from build123d import *

# Parameters (mm, degrees)
SKETCH1_W           = 170
SKETCH1_H           = 216
BOSS_EXTRUDE1_DEPTH = 5
SKETCH2_R           = 1.5
CUT_EXTRUDE1_DEPTH  = 138.528178931
SKETCH9_W           = 170
SKETCH9_H           = 90
BOSS_EXTRUDE2_DEPTH = 3
SKETCH10_W          = 219
SKETCH10_H          = 90
BOSS_EXTRUDE3_DEPTH = 5
BOSS_EXTRUDE5_START = 5
SKETCH11_W          = 219
SKETCH11_H          = 90
BOSS_EXTRUDE5_DEPTH = 5
SKETCH14_W          = 180
SKETCH14_H          = 90
CUT_EXTRUDE2_DEPTH  = 3
SKETCH15_W          = 180
SKETCH15_H          = 90
BOSS_EXTRUDE6_DEPTH = 5


with BuildPart() as part:
    # Sketch1 → Boss-Extrude1 (new body)
    with BuildSketch(Plane(origin=(0, 0, 0), x_dir=(1, 0, 0), z_dir=(0, 1, 0))):
        Rectangle(SKETCH1_W, SKETCH1_H)
    extrude(amount=BOSS_EXTRUDE1_DEPTH)

    # Sketch2 → Cut-Extrude1 (cut, through all)
    with BuildSketch(Plane(origin=(0, 5, 0), x_dir=(1, 0, 0), z_dir=(0, 1, 0))):
        with Locations(Location((-75, 98, 0), (0, 0, 270))):
            Circle(SKETCH2_R)
        with Locations(Location((75, 98, 0), (0, 0, 270))):
            Circle(SKETCH2_R)
        with Locations(Location((-75, -98, 0), (0, 0, 270))):
            Circle(SKETCH2_R)
        with Locations(Location((75, -98, 0), (0, 0, 270))):
            Circle(SKETCH2_R)
    extrude(amount=-CUT_EXTRUDE1_DEPTH, mode=Mode.SUBTRACT)

    # Sketch9 → Boss-Extrude2 (add)
    with BuildSketch(Plane(origin=(0, 0, -108), x_dir=(-1, 0, 0), z_dir=(0, 0, -1))):
        with Locations((0, 45)):
            Rectangle(SKETCH9_W, SKETCH9_H)
    extrude(amount=BOSS_EXTRUDE2_DEPTH)

    # Sketch10 → Boss-Extrude3 (add)
    with BuildSketch(Plane(origin=(85, 0, 0), x_dir=(0, 0, -1), z_dir=(1, 0, 0))):
        with Locations((1.5, 45)):
            Rectangle(SKETCH10_W, SKETCH10_H)
        with BuildLine():
            Line((-84, 5), (-41, 5))
            Line((-41, 5), (-41, 44))
            ThreePointArc((-41, 44), (-41.878679656, 46.121320344), (-44, 47))
            Line((-44, 47), (-81, 47))
            ThreePointArc((-81, 47), (-83.121320344, 46.121320344), (-84, 44))
            Line((-84, 44), (-84, 5))
        make_face(mode=Mode.SUBTRACT)
        with BuildLine():
            Line((84, 5), (41, 5))
            Line((41, 5), (41, 44))
            ThreePointArc((41, 44), (41.878679656, 46.121320344), (44, 47))
            Line((44, 47), (81, 47))
            ThreePointArc((81, 47), (83.121320344, 46.121320344), (84, 44))
            Line((84, 44), (84, 5))
        make_face(mode=Mode.SUBTRACT)
    extrude(amount=BOSS_EXTRUDE3_DEPTH)

    # Sketch11 → Boss-Extrude5 (add)
    with BuildSketch(Plane.ZY.offset(85).offset(BOSS_EXTRUDE5_START)):
        with Locations((-1.5, 45)):
            Rectangle(SKETCH11_W, SKETCH11_H)
        with BuildLine():
            Line((-84, 5), (-84, 44))
            ThreePointArc((-84, 44), (-83.121320344, 46.121320344), (-81, 47))
            Line((-81, 47), (-44, 47))
            ThreePointArc((-44, 47), (-41.878679656, 46.121320344), (-41, 44))
            Line((-41, 44), (-41, 5))
            Line((-41, 5), (-84, 5))
        make_face(mode=Mode.SUBTRACT)
        with BuildLine():
            Line((41, 5), (41, 44))
            ThreePointArc((41, 44), (41.878679656, 46.121320344), (44, 47))
            Line((44, 47), (81, 47))
            ThreePointArc((81, 47), (83.121320344, 46.121320344), (84, 44))
            Line((84, 44), (84, 5))
            Line((84, 5), (41, 5))
        make_face(mode=Mode.SUBTRACT)
    extrude(amount=-BOSS_EXTRUDE5_DEPTH)

    # Sketch14 → Cut-Extrude2 (cut)
    with BuildSketch(Plane(origin=(0, 0, -111), x_dir=(-1, 0, 0), z_dir=(0, 0, -1))):
        with Locations((0, 45)):
            Rectangle(SKETCH14_W, SKETCH14_H)
    extrude(amount=-CUT_EXTRUDE2_DEPTH, mode=Mode.SUBTRACT)

    # Sketch15 → Boss-Extrude6 (add)
    with BuildSketch(Plane.XY.offset(108)):
        with Locations((0, 45)):
            Rectangle(SKETCH15_W, SKETCH15_H)
    extrude(amount=BOSS_EXTRUDE6_DEPTH)


solid = part.part
Geometry: final body of the model. Coordinates: model frame, mm. A direction names the side the tool comes from. Give positions to 0.01 mm unless a question says otherwise; leave off trailing zeros. Write each loop counter-clockwise with the first axis right and the second up, starting at its lowest first coordinate (ties: lowest second). Pieces come first, ordered by that corner, then holes.
(1) Cut plane A-A, the plane y = 11. Return loops of the section in (x, z).
(2) Cut plane D-D, the plane x = -35.5. Return loops of the section in (y, z), then the cut area to 3 significant figures.
(3) Cut plane C-C, the plane z = 29. Return loops of the section in (x, y).
(4) Cut plane B-B, the plane y = 66. Return loops of the section in (x, z), then the cut area to 3 significant figures.
(5) Access query for faces 1 (the flat face through (87, 25, 84)), 2 (the flat face through (-1, 46, 113)), 3 (the flat face through (-1, 48, 108)). Directions: +Z, -Z, +X, -X, +Y, -Y. A direction counts if a zero-diameter tool reaches every point of the face in a straight line with its end or side. Return the directions, or none.
(6) Mould query, pull axis X, two halves, no side actions, for faces 4 (the flat face through (-88, 25, 84)), 5 (the flat face through (-1, 5, 2)), 6 (the flat face through (90, 44, 1)), 7 (the flat face through (85, 58, 2)). Classes: released by +X, released by -X, zero draft, split by the parting line, or undercut.
(7) Ray query, line 1 (Z direction, x = -75, y = 2); line 2 (X direction, y = 1, z = -98); line 3 (X direction, y = 19, z = -3.5). Return the intervals inside material, ascending.
(8) First-contact query: P1, Ø3, axis at x = -55.5, z = -30.5, coming from the +Y side; P2, Ø1.8, axis at x = -75, z = -98, coming from the +Y side. Flat tips, straight axial feed; report the tip coordinate or a pass-through.
Values follow:
1. outline: (-90, -108) - (-85, -108) - (-85, -84) - (-90, -84) - close; (-90, -41) - (-85, -41) - (-85, 41) - (-90, 41) - close; (-90, 84) - (-85, 84) - (-85, 108) - (85, 108) - (85, 84) - (90, 84) - (90, 113) - (-90, 113) - close; (85, -108) - (90, -108) - (90, -84) - (85, -84) - close; (85, -41) - (90, -41) - (90, 41) - (85, 41) - close
2. outline: (0, -108) - (5, -108) - (5, 108) - (90, 108) - (90, 113) - (0, 113) - close
2. area: 1,530 mm2
3. outline: (-90, 0) - (90, 0) - (90, 90) - (85, 90) - (85, 5) - (-85, 5) - (-85, 90) - (-90, 90) - close
4. outline: (-90, -108) - (-85, -108) - (-85, 108) - (85, 108) - (85, -108) - (90, -108) - (90, 113) - (-90, 113) - close
4. area: 3,060 mm2
5. face 1: +X, -X
5. face 2: +Z, +X, -X, +Y, -Y
5. face 3: -Z, +Y
6. face 4: zero draft
6. face 5: undercut
6. face 6: released by +X
6. face 7: undercut
7. line 1: z = -108 to -99.5, -96.5 to 96.5, 99.5 to 113
7. line 2: x = -90 to -76.5, -73.5 to 73.5, 76.5 to 90
7. line 3: x = -90 to -85, 85 to 90
8. P1: stops at y = 5
8. P2: passes through
